from build123d import *

# Parameters (mm, degrees)
SKETCH_1_W        = 50
SKETCH_1_H        = 13.8
SKETCH_1_R        = 2.5
EXTRUDE_1_DEPTH   = 15
EXTRUDE_1_2_DEPTH = 15
EXTRUDE_START     = -4
SKETCH_2_R        = 15
EXTRUDE_2_DEPTH   = 8
SKETCH_3_R        = 4
EXTRUDE_3_DEPTH   = 57.6
EXTRUDE_4_DEPTH   = 10


with BuildPart() as part:
    # Sketch 1 → Extrude 1 (new, symmetric)
    with BuildSketch(Plane(origin=(0, 0, 0), x_dir=(1, 0, 0), z_dir=(0, 1, 0))):
        with Locations((0, 10.9)):
            Rectangle(SKETCH_1_W, SKETCH_1_H)
        with Locations(Location((-19, 10.9, 0), (0, 0, 270))):
            Circle(SKETCH_1_R, mode=Mode.SUBTRACT)
        with Locations(Location((19, 10.9, 0), (0, 0, 270))):
            Circle(SKETCH_1_R, mode=Mode.SUBTRACT)
    extrude(amount=EXTRUDE_1_DEPTH, both=True)



with BuildPart() as body_2:
    # Sketch 1 → Extrude 1 2 (new, symmetric)
    with BuildSketch(Plane(origin=(0, 0, 0), x_dir=(1, 0, 0), z_dir=(0, 1, 0))):
        with Locations((0, -10.9)):
            Rectangle(SKETCH_1_W, SKETCH_1_H)
        with Locations(Location((15, -10.9, 0), (0, 0, 270))):
            Circle(SKETCH_1_R, mode=Mode.SUBTRACT)
        with Locations(Location((-15, -10.9, 0), (0, 0, 270))):
            Circle(SKETCH_1_R, mode=Mode.SUBTRACT)
    extrude(amount=EXTRUDE_1_2_DEPTH, both=True)


with BuildPart() as part_1:
    add(part.part)

    add(body_2.part)  # Extrude 2 merges body 2
    # Sketch 2 → Extrude 2 (add)
    with BuildSketch(Plane.XY.offset(EXTRUDE_START)):
        with Locations(Location((0, 0, 0), (0, 0, 90))):
            Circle(SKETCH_2_R)
    extrude(amount=EXTRUDE_2_DEPTH)

    # Sketch 3 → Extrude 3 (add)
    with BuildSketch(Plane.XY.offset(22.8)):
        Circle(SKETCH_3_R)
    extrude(amount=-EXTRUDE_3_DEPTH)

    # Sketch 4 → Extrude 4 (add)
    with BuildSketch(Plane(origin=(0, 0, -17.8), x_dir=(-1, 0, 0), z_dir=(0, 0, -1))):
        Polygon((-10.021943358, 0), (-5.010971679, -8.679257543), (5.010971679, -8.679257543), (10.021943358, 0), (5.010971679, 8.679257543), (-5.010971679, 8.679257543), align=None)
    extrude(amount=EXTRUDE_4_DEPTH)


solid = part_1.part
Design review of the part built by this model. Coordinates are the model's own, in mm. A direction names the side the tool comes from. Give positions to 0.01 mm unless a question says otherwise; leave off trailing zeros. Loops run counter-clockwise (first coordinate to the right, second up) from the corner with the lowest first, then second, coordinate; pieces in that order, holes last. Notation, with made-up numbers: (80.5, 29.25) - (126.5, 29.25) arc R26 ccw to (126.5, 48.25) - close; hole circle Ø11 at (-2.5, 13.5). An arc over 180 degrees is marked (long way). Write item = value, one per line.
1) Clearance check with flat-ended pins moving along their axes: pin 1 Ø3 at (x, z) = (-1, -21) entering from -Y; pin 2 Ø7.5 at (x, y) = (-10.5, -1.5) entering from +Z; pin 3 Ø7.5 at (x, y) = (7, -5) entering from -Z. State where each tip first meets the part, or that it passes through.
Result sheet:
pin_1 = -8.68
pin_2 = 17.8
pin_3 = -27.8
2) Draft analysis for pull direction Z (two halves, no side actions). For faces 4 (the face through (-4.3, 0.1, -27.8)), 5 (the face through (0, -15, -11)), 6 (the face through (-18, 0, 4)), state which applies: +Z half, -Z half, draft (parallel to the pull), parting line (faces both ways), or undercut.
Result sheet:
face_4 = -Z half
face_5 = draft
face_6 = undercut
3) Take a section at C-C on z = -11.5. State the section outline as (x, y) points.
Result sheet:
outline = (-25, -15) - (-21.43, -15) - (-21.43, 15) - (-25, 15) - close; (-16.57, -15) - (16.57, -15) - (16.57, 15) - (-16.57, 15) - close; (21.43, -15) - (25, -15) - (25, 15) - (21.43, 15) - close
4) Take a section at A-A on x = 19. State the section outline as (y, z) points, and give its area (3 significant figures).
Result sheet:
outline = (-15, -17.8) - (15, -17.8) - (15, -13.4) - (-15, -13.4) - close; (-15, -8.4) - (15, -8.4) - (15, -4) - (-15, -4) - close; (-15, 4) - (15, 4) - (15, 17.8) - (-15, 17.8) - close
area = 678 mm2
5) To check wall thickness, follow line 1 (X direction, y = -3.75, z = -10.9); line 2 (X direction, y = -2.5, z = 10.9); line 3 (Z direction, x = -20, y = -11.5). State the ranges of each line that lie inside material, in increasing order.
Result sheet:
line_1 = -25 to -21.5, -16.5 to 16.5, 21.5 to 25
line_2 = -25 to -17.5, -12.5 to 12.5, 17.5 to 25
line_3 = -17.8 to -13.19, -8.61 to -4, 4 to 17.8
6) Take a section at D-D on z = -30.5. State the section outline as (x, y) points.
Result sheet:
outline = circle Ø8 at (0, 0)
7) Take a section at B-B on y = -7. State the section outline as (x, z) points.
Result sheet:
outline = (-25, -17.8) - (-5.98, -17.8) - (-5.98, -27.8) - (5.98, -27.8) - (5.98, -17.8) - (25, -17.8) - (25, -4) - (13.27, -4) - (13.27, 4) - (25, 4) - (25, 17.8) - (-25, 17.8) - (-25, 4) - (-13.27, 4) - (-13.27, -4) - (-25, -4) - close; hole circle Ø5 at (-19, -10.9); hole circle Ø5 at (-15, 10.9); hole circle Ø5 at (15, 10.9); hole circle Ø5 at (19, -10.9)
8) Tool access review of faces 1 (the face through (7.48, 4.4, -22.73)), 2 (the face through (-0.66, -14.985, -0.056)), 3 (the face through (-0.867, -3.905, -31.251)): name each direction out of +Z, -Z, +X, -X, +Y, -Y from which nothing blocks a thin tool from reaching the whole face with its end or side.
Result sheet:
face_1 = -Z, +X, +Y
face_2 = none
face_3 = -Z
